Verification items for this drawing (mm, ordinates from the low corner). A direction names the side the tool comes from. Round coordinates to 2 decimals unless told otherwise and drop trailing zeros. Order: outer loops, then holes, each group sorted by start corner. A loop starts at its lowest first (then second) coordinate and runs counter-clockwise, first axis right, second up. Notation, with made-up numbers: (-21, 39) -> (-8, 39) arc R6 ccw to (-8, 43) -> close; hole circle Ø11 at (82, 72). An arc over 180 degrees is marked (long way). Use a Markdown table: item, result. Add a question column.
Item 1: Sectioned sample at A-A, the plane z = 12.5. Record the cut outline in (x, y).
Item 2: Gauge pin test, flat ends, axial feed: pin 1 Ø2.5 at (x, z) = (8, 16.07) entering from +Y; pin 2 Ø15 at (x, y) = (16.5, 37) entering from +Z; pin 3 Ø2.5 at (x, y) = (15, 20.14) entering from +Z. Record the tip position at first contact, or that the pin passes through.
Item 3: Sectioned sample at B-B, the plane x = 15. Record the cut outline in (y, z).
Item 4: Set-up check for the marked faces 4 and 5: record each of +Z, -Z, +X, -X, +Y, -Y from which the full face is reachable in a straight line by a thin tool's end or side.
Item 5: Mould release check, pull along Y, two halves, no side actions. Record for the marked faces 1, 2 and 3: pulls with the +Y half, pulls with the -Y half, needs draft (parallel to the pull), parting line crosses it, or undercut.
Item 6: Sectioned sample at C-C, the plane x = 25. Record the cut outline in (y, z).
Item 7: Sectioned sample at D-D, the plane y = 26.5. Record the cut outline in (x, z).
Item 8: Material ranges on probe 1 along Y at (x, z) = (12.75, 5); probe 2 along Y at (x, z) = (15, 1.15) (1 decimal); probe 3 along Z at (x, y) = (14, 35.5), recorded low to high. Write a range as [from, to].
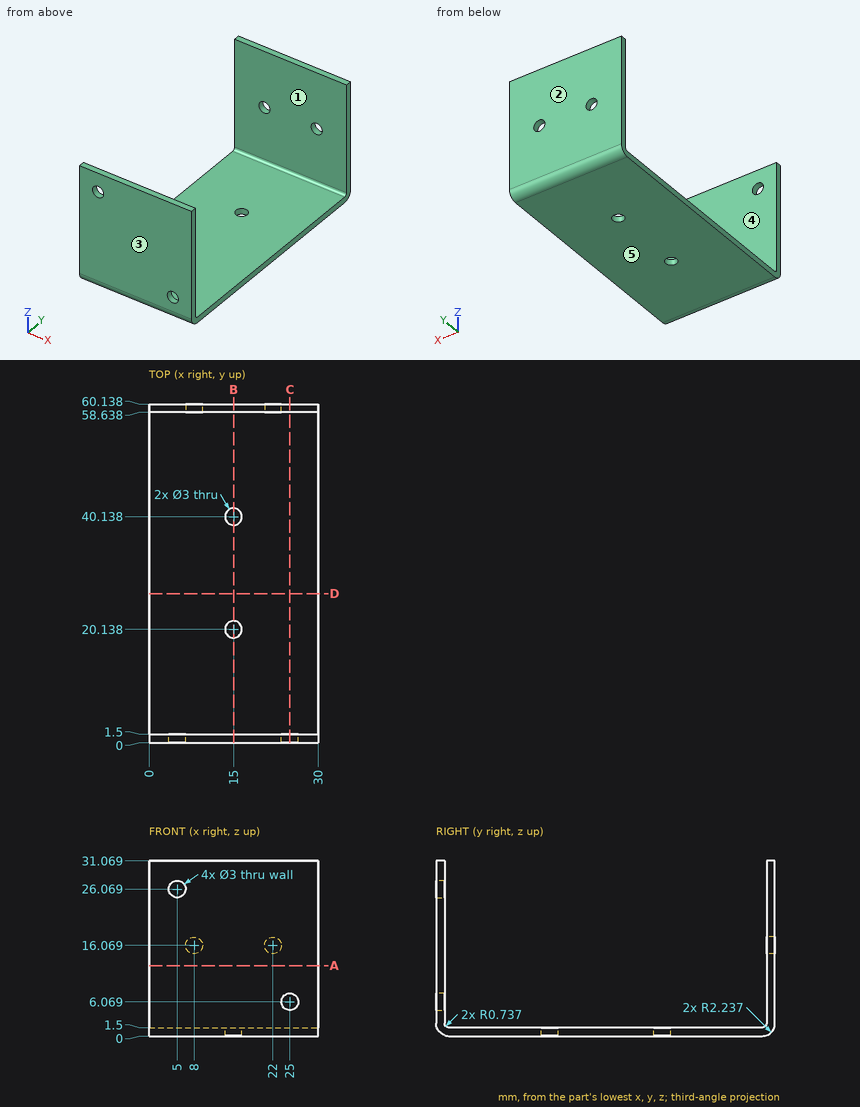
Found:
| question | item | result |
|---|---|---|
| 1 | outline | (0, 0) -> (30, 0) -> (30, 1.5) -> (0, 1.5) -> close; (0, 58.64) -> (30, 58.64) -> (30, 60.14) -> (0, 60.14) -> close |
| 2 | pin 1 | stops at y = 1.5 |
| 2 | pin 2 | stops at z = 1.5 |
| 2 | pin 3 | passes through |
| 3 | outline | (0, 2.24) arc R2.24 ccw to (2.24, 0) -> (18.64, 0) -> (18.64, 1.5) -> (2.24, 1.5) arc R0.74 cw to (1.5, 2.24) -> (1.5, 31.07) -> (0, 31.07) -> close; (21.64, 0) -> (38.64, 0) -> (38.64, 1.5) -> (21.64, 1.5) -> close; (41.64, 0) -> (57.9, 0) arc R2.24 ccw to (60.14, 2.24) -> (60.14, 31.07) -> (58.64, 31.07) -> (58.64, 2.24) arc R0.74 cw to (57.9, 1.5) -> (41.64, 1.5) -> close |
| 4 | face 4 | +Z, +X, -X |
| 4 | face 5 | -Z, +X, -X, +Y, -Y |
| 5 | face 1 | undercut |
| 5 | face 2 | pulls with the +Y half |
| 5 | face 3 | pulls with the -Y half |
| 6 | outline | (0, 2.24) arc R2.24 ccw to (2.24, 0) -> (57.9, 0) arc R2.24 ccw to (60.14, 2.24) -> (60.14, 31.07) -> (58.64, 31.07) -> (58.64, 2.24) arc R0.74 cw to (57.9, 1.5) -> (2.24, 1.5) arc R0.74 cw to (1.5, 2.24) -> (1.5, 4.57) -> (0, 4.57) -> close; (0, 7.57) -> (1.5, 7.57) -> (1.5, 31.07) -> (0, 31.07) -> close |
| 7 | outline | (0, 0) -> (30, 0) -> (30, 1.5) -> (0, 1.5) -> close |
| 8 | probe 1 | y = [0, 1.5], [58.64, 60.14] |
| 8 | probe 2 | y = [0.3, 18.6], [21.6, 38.6], [41.6, 59.9] |
| 8 | probe 3 | z = [0, 1.5] |
